from build123d import *

# Parameters (mm, degrees)
SKETCH_1_R      = 1.5
SKETCH_1_R_2    = 11.5
SKETCH_1_R_3    = 2
EXTRUDE_1_DEPTH = 2
FILLET_1_R      = 1.3


with BuildPart() as part:
    # 草图1 → 凸台-拉伸1 (new body)
    with BuildSketch(Plane.XY):
        Polygon((22.5, -27), (-22.5, -27), (-27.5, -27), (-27.5, -23), (-22.5, -23), (-22.5, -17.05), (-18.5, -17.05), (-18.5, -18.5), (-15.3, -18.5), (-15.3, -17.05), (-12.1, -17.05), (-12.1, -12.95), (-15.3, -12.95), (-15.3, -11.5), (-18.5, -11.5), (-18.5, -12.95), (-22.5, -12.95), (-22.5, -4), (-27.5, -4), (-27.5, 4), (-22.5, 4), (-22.5, 12.95), (-18.5, 12.95), (-18.5, 11.5), (-15.3, 11.5), (-15.3, 12.95), (-12.1, 12.95), (-12.1, 17.05), (-15.3, 17.05), (-15.3, 18.5), (-18.5, 18.5), (-18.5, 17.05), (-22.5, 17.05), (-22.5, 23), (-27.5, 23), (-27.5, 27), (-22.5, 27), (-9, 27), (-9, 41), (-22, 41), (-22, 53), (22, 53), (22, 41), (9, 41), (9, 27), (22.5, 27), (27.5, 27), (27.5, 23), (22.5, 23), (22.5, 17.05), (18.5, 17.05), (18.5, 18.5), (15.3, 18.5), (15.3, 17.05), (12.1, 17.05), (12.1, 12.95), (15.3, 12.95), (15.3, 11.5), (18.5, 11.5), (18.5, 12.95), (22.5, 12.95), (22.5, 4), (27.5, 4), (27.5, -4), (22.5, -4), (22.5, -12.95), (18.5, -12.95), (18.5, -11.5), (15.3, -11.5), (15.3, -12.95), (12.1, -12.95), (12.1, -17.05), (15.3, -17.05), (15.3, -18.5), (18.5, -18.5), (18.5, -17.05), (22.5, -17.05), (22.5, -23), (27.5, -23), (27.5, -27), align=None)
        with Locations((9.899494937, 9.899494937)):
            Circle(SKETCH_1_R, mode=Mode.SUBTRACT)
        Circle(SKETCH_1_R_2, mode=Mode.SUBTRACT)
        with Locations((9.899494937, -9.899494937)):
            Circle(SKETCH_1_R, mode=Mode.SUBTRACT)
        with Locations((-9.899494937, -9.899494937)):
            Circle(SKETCH_1_R, mode=Mode.SUBTRACT)
        with Locations((-9.899494937, 9.899494937)):
            Circle(SKETCH_1_R, mode=Mode.SUBTRACT)
        with Locations((-18, 47)):
            Circle(SKETCH_1_R_3, mode=Mode.SUBTRACT)
        with Locations((18, 47)):
            Circle(SKETCH_1_R_3, mode=Mode.SUBTRACT)
        with Locations((0, 29)):
            Circle(SKETCH_1_R_3, mode=Mode.SUBTRACT)
    extrude(amount=EXTRUDE_1_DEPTH)

    # 圆角1
    fillet_1_edges = [part.edges().sort_by_distance(p)[0] for p in [
        (-9, 27, 1),
        (-9, 41, 1),
        (-22, 41, 1),
        (-22, 53, 1),
        (22, 53, 1),
        (22, 41, 1),
        (9, 41, 1),
        (9, 27, 1),
        (27.5, 23, 1),
        (27.5, 4, 1),
        (27.5, -4, 1),
        (27.5, -23, 1),
        (-27.5, -23, 1),
        (-27.5, -4, 1),
        (-27.5, 4, 1),
        (-27.5, 23, 1),
    ]]
    fillet(fillet_1_edges, radius=FILLET_1_R)


solid = part.part
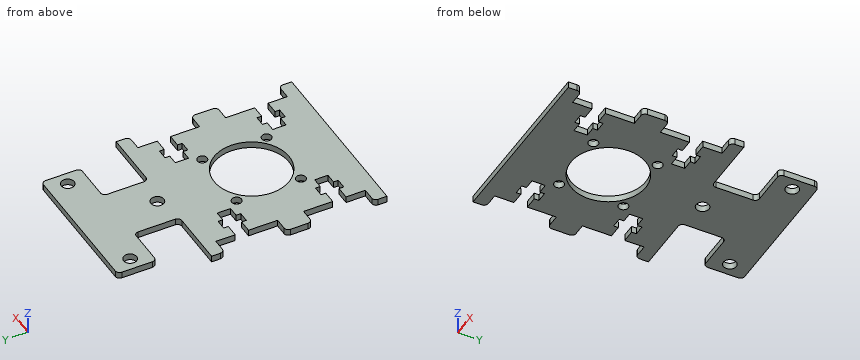
Geometry: final body of the model. Coordinates: model frame, mm. Round coordinates to 2 decimals unless told otherwise and drop trailing zeros. Loops run counter-clockwise (first coordinate to the right, second up) from the corner with the lowest first, then second, coordinate; pieces in that order, holes last.
Q1. Section B-B on y = 0. Return loops of the section in (x, z), plus the area to 3 significant figures.
Q2. Material intervals for L1, parallel to Y at x = 0, z = 1.25; L2, parallel to Y at x = 18, z = 1.05; L3, parallel to Y at x = -25, z = 0.45, sorted ascending.
Q3. Pin query (flat end, axial travel): P1, Ø0.6, axis at y = -6.5, z = 1.5, coming from the +X side; P2, Ø5, axis at x = 9.9, y = 9.9, coming from the +Z side; P3, Ø0.6, axis at y = 8.5, z = 0.5, coming from the -X side; P4, Ø0.6, axis at y = 14.5, z = 0.5, coming from the +X side. Return the tip coordinate at first contact, or that it passes through.
Q4. Section D-D on z = 1.5. State how many separate pieces and enclosed holes the cut face has, plus the area to 3 significant figures.
Q5. Section C-C on y = 48. Return loops of the section in (x, z), plus the area to 3 significant figures.
Q6. Section A-A on x = 0. Return loops of the section in (y, z), plus the area to 3 significant figures.
Evaluation:
1. outline: (-27.5, 0) - (-11.5, 0) - (-11.5, 2) - (-27.5, 2) - close; (11.5, 0) - (27.5, 0) - (27.5, 2) - (11.5, 2) - close
1. area: 64.0 mm2
2. L1: y = -27 to -11.5, 11.5 to 27, 31 to 53
2. L2: y = -27 to -18.5, -11.5 to 11.5, 18.5 to 27, 41 to 45, 49 to 53
2. L3: y = -27 to -23, -4 to 4, 23 to 27
3. P1: stops at x = 22.5
3. P2: stops at z = 2
3. P3: stops at x = -22.5
3. P4: stops at x = 12.1
4. separate pieces: 1
4. enclosed holes: 8
4. area: 2,680 mm2
5. outline: (-22, 0) - (-19.73, 0) - (-19.73, 2) - (-22, 2) - close; (-16.27, 0) - (16.27, 0) - (16.27, 2) - (-16.27, 2) - close; (19.73, 0) - (22, 0) - (22, 2) - (19.73, 2) - close
5. area: 74.1 mm2
6. outline: (-27, 0) - (-11.5, 0) - (-11.5, 2) - (-27, 2) - close; (11.5, 0) - (27, 0) - (27, 2) - (11.5, 2) - close; (31, 0) - (53, 0) - (53, 2) - (31, 2) - close
6. area: 106 mm2
